```python
from build123d import *

# Parameters (mm, degrees)
SKETCH1_W           = 44.362146026
SKETCH1_H           = 10
BOSS_EXTRUDE1_DEPTH = 8
SKETCH2_R           = 1.6
CUT_EXTRUDE1_DEPTH  = 52.107729357
CUT_EXTRUDE2_START  = -17.925297
SKETCH3_R           = 3.05
CUT_EXTRUDE2_DEPTH  = 12.925297
FILLET1_R           = 2


with BuildPart() as part:
    # Sketch1 → Boss-Extrude1 (new body)
    with BuildSketch(Plane.XY):
        with BuildLine():
            Line((-29.953929645, -23), (-37.509998667, -23))
            ThreePointArc((-37.509998667, -23), (-35.812927639, -25.562359318), (-33.941125497, -28))
            Line((-33.941125497, -28), (-22.181073013, -28))
            Line((-22.181073013, -28), (-22.181073013, -23))
            Line((-22.181073013, -23), (-29.953929645, -23))
        make_face()
        with BuildLine():
            Line((-37.509998667, -23), (-43.266615306, -23))
            ThreePointArc((-43.266615306, -23), (0, -49), (43.266615306, -23))
            Line((43.266615306, -23), (37.509998667, -23))
            ThreePointArc((37.509998667, -23), (35.812927639, -25.562359318), (33.941125497, -28))
            ThreePointArc((33.941125497, -28), (28.503075122, -33.519765939), (22.181073013, -38))
            ThreePointArc((22.181073013, -38), (0, -44), (-22.181073013, -38))
            ThreePointArc((-22.181073013, -38), (-28.503075122, -33.519765939), (-33.941125497, -28))
            ThreePointArc((-33.941125497, -28), (-35.812927639, -25.562359318), (-37.509998667, -23))
        make_face()
        with BuildLine():
            Line((-22.181073013, -28), (-33.941125497, -28))
            ThreePointArc((-33.941125497, -28), (-28.503075122, -33.519765939), (-22.181073013, -38))
            Line((-22.181073013, -38), (-22.181073013, -28))
        make_face()
        with BuildLine():
            ThreePointArc((22.181073013, -38), (28.503075122, -33.519765939), (33.941125497, -28))
            Line((33.941125497, -28), (22.181073013, -28))
            Line((22.181073013, -28), (22.181073013, -38))
        make_face()
        with BuildLine():
            ThreePointArc((33.941125497, -28), (35.812927639, -25.562359318), (37.509998667, -23))
            Line((37.509998667, -23), (22.181073013, -23))
            Line((22.181073013, -23), (22.181073013, -28))
            Line((22.181073013, -28), (33.941125497, -28))
        make_face()
        with Locations((0, -33)):
            Rectangle(SKETCH1_W, SKETCH1_H)
        with BuildLine():
            Line((22.181073013, -38), (-22.181073013, -38))
            ThreePointArc((-22.181073013, -38), (0, -44), (22.181073013, -38))
        make_face()
    extrude(amount=BOSS_EXTRUDE1_DEPTH)

    # Sketch2 → Cut-Extrude1 (cut, through all)
    with BuildSketch(Plane(origin=(0, -23, 0), x_dir=(1, 0, 0), z_dir=(0, 1, 0))):
        with Locations(Location((-29.996615306, -4, 0), (0, 0, 270))):
            Circle(SKETCH2_R)
    cut_extrude1 = extrude(amount=-CUT_EXTRUDE1_DEPTH, mode=Mode.SUBTRACT)

    # Sketch3 → Cut-Extrude2 (cut)
    with BuildSketch(Plane(origin=(0, -23, 0), x_dir=(1, 0, 0), z_dir=(0, 1, 0)).offset(CUT_EXTRUDE2_START)):
        with Locations(Location((-29.996615306, -4, 0), (0, 0, 90))):
            Circle(SKETCH3_R)
    cut_extrude2 = extrude(amount=CUT_EXTRUDE2_DEPTH, mode=Mode.SUBTRACT)

    # Mirror1: Cut-Extrude1, Cut-Extrude2 across plane
    add(cut_extrude1.mirror(Plane(origin=(0, 0, 0), x_dir=(0, 0, 1), z_dir=(1, 0, 0))), mode=Mode.SUBTRACT)
    add(cut_extrude2.mirror(Plane(origin=(0, 0, 0), x_dir=(0, 0, 1), z_dir=(1, 0, 0))), mode=Mode.SUBTRACT)

    # Fillet1
    # the kernel refuses this fillet: 2 mm, written as the material it takes off along each edge
    with BuildSketch(Plane(origin=(22.181073013, -28, 8), x_dir=(0, -1, 0), z_dir=(-1, 0, 0))) as fillet1_piece_1:
        with BuildLine():
            CenterArc((FILLET1_R, -FILLET1_R), FILLET1_R, 90, 90)
            Line((0, -FILLET1_R), (0, 0))
            Line((0, 0), (FILLET1_R, 0))
        make_face()
    extrude(amount=44.362146026, mode=Mode.SUBTRACT)
    with BuildSketch(Plane(origin=(22.181073013, -28, 0), x_dir=(0, -1, 0), z_dir=(-1, 0, 0))) as fillet1_piece_2:
        with BuildLine():
            CenterArc((FILLET1_R, FILLET1_R), FILLET1_R, 180, 90)
            Line((0, FILLET1_R), (0, 0))
            Line((0, 0), (FILLET1_R, 0))
        make_face()
    extrude(amount=44.362146026, mode=Mode.SUBTRACT)
    with BuildSketch(Plane(origin=(22.181073013, -18, 0), x_dir=(1, 0, 0), z_dir=(0, -1, 0))) as fillet1_piece_3:
        with BuildLine():
            CenterArc((FILLET1_R, FILLET1_R), FILLET1_R, 180, 90)
            Line((0, FILLET1_R), (0, 0))
            Line((0, 0), (FILLET1_R, 0))
        make_face()
    extrude(amount=10, mode=Mode.SUBTRACT)
    with BuildSketch(Plane(origin=(-22.181073013, -28, 8), x_dir=(-1, 0, 0), z_dir=(0, 1, 0)), Plane(origin=(22.181073013, -18, 8), x_dir=(1, 0, 0), z_dir=(0, -1, 0)), Plane(origin=(-22.181073013, -28, 0), x_dir=(0, 0, 1), z_dir=(0, 1, 0))) as fillet1_piece_4:
        with BuildLine():
            CenterArc((FILLET1_R, -FILLET1_R), FILLET1_R, 90, 90)
            Line((0, -FILLET1_R), (0, 0))
            Line((0, 0), (FILLET1_R, 0))
        make_face()
    extrude(amount=10, mode=Mode.SUBTRACT)
    with BuildSketch(Plane(origin=(-17.181073013, -23, 8), x_dir=(0, -1, 0), z_dir=(-1, 0, 0)), Plane(origin=(48.266615306, -23, 8), x_dir=(0, -1, 0), z_dir=(-1, 0, 0)), Plane(origin=(-48.266615306, -23, 0), x_dir=(0, -1, 0), z_dir=(1, 0, 0))) as fillet1_piece_5:
        with BuildLine():
            CenterArc((FILLET1_R, -FILLET1_R), FILLET1_R, 90, 90)
            Line((0, -FILLET1_R), (0, 0))
            Line((0, 0), (FILLET1_R, 0))
        make_face()
    extrude(amount=31.085542293, mode=Mode.SUBTRACT)
    with BuildSketch(Plane(origin=(0, 0, 8), x_dir=(-0.9262421127905929, -0.3769291027411106, 0), z_dir=(-0.3769291027411106, 0.9262421127905929, 0))) as fillet1_piece_6:
        with BuildLine():
            CenterArc((49 - FILLET1_R, -FILLET1_R), FILLET1_R, 0, 90)
            Line((49, -FILLET1_R), (49, 0))
            Line((49, 0), (49 - FILLET1_R, 0))
        make_face()
    revolve(axis=Axis((0, 0, 8), (0, 0, 1)), revolution_arc=135.712813104, mode=Mode.SUBTRACT)
    with BuildSketch(Plane(origin=(48.266615306, -23, 0), x_dir=(0, -1, 0), z_dir=(-1, 0, 0))) as fillet1_piece_7:
        with BuildLine():
            CenterArc((FILLET1_R, FILLET1_R), FILLET1_R, 180, 90)
            Line((0, FILLET1_R), (0, 0))
            Line((0, 0), (FILLET1_R, 0))
        make_face()
    extrude(amount=31.085542293, mode=Mode.SUBTRACT)
    with BuildSketch(Plane(origin=(0, 0, 0), x_dir=(-0.9262421127905929, -0.3769291027411106, 0), z_dir=(-0.3769291027411106, 0.9262421127905929, 0))) as fillet1_piece_8:
        with BuildLine():
            CenterArc((49 - FILLET1_R, FILLET1_R), FILLET1_R, 270, 90)
            Line((49, FILLET1_R), (49, 0))
            Line((49, 0), (49 - FILLET1_R, 0))
        make_face()
    revolve(axis=Axis((0, 0, 0), (0, 0, 1)), revolution_arc=135.712813104, mode=Mode.SUBTRACT)
    with BuildSketch(Plane(origin=(22.181073013, -18, 8), x_dir=(1, 0, 0), z_dir=(0, -1, 0))) as fillet1_piece_9a_section:
        with BuildLine():
            CenterArc((FILLET1_R, -FILLET1_R), FILLET1_R, 90, 90)
            Line((0, -FILLET1_R), (0, 0))
            Line((0, 0), (FILLET1_R, 0))
        make_face()
    fillet1_piece_9a = extrude(amount=15, mode=Mode.PRIVATE)
    fillet1_piece_9a = split(fillet1_piece_9a, bisect_by=Plane(origin=(22.633863241, -28, 7.547209771), z_dir=(0, -1, 0)), keep=Keep.TOP, mode=Mode.PRIVATE)
    with BuildSketch(Plane(origin=(27.181073013, -28, 8), x_dir=(0, -1, 0), z_dir=(-1, 0, 0))) as fillet1_piece_9b_section:
        with BuildLine():
            CenterArc((FILLET1_R, -FILLET1_R), FILLET1_R, 90, 90)
            Line((0, -FILLET1_R), (0, 0))
            Line((0, 0), (FILLET1_R, 0))
        make_face()
    fillet1_piece_9b = extrude(amount=49.362146026, mode=Mode.PRIVATE)
    fillet1_piece_9b = split(fillet1_piece_9b, bisect_by=Plane(origin=(22.181073013, -28.452790229, 7.547209771), z_dir=(1, 0, 0)), keep=Keep.TOP, mode=Mode.PRIVATE)
    fillet1_piece_9 = fillet1_piece_9a & fillet1_piece_9b
    add(fillet1_piece_9, mode=Mode.SUBTRACT)
    with BuildSketch(Plane(origin=(22.181073013, -28, 8), x_dir=(0, -1, 0), z_dir=(-1, 0, 0))) as fillet1_piece_10a_section:
        with BuildLine():
            CenterArc((FILLET1_R, -FILLET1_R), FILLET1_R, 90, 90)
            Line((0, -FILLET1_R), (0, 0))
            Line((0, 0), (FILLET1_R, 0))
        make_face()
    fillet1_piece_10a = extrude(amount=49.362146026, mode=Mode.PRIVATE)
    fillet1_piece_10a = split(fillet1_piece_10a, bisect_by=Plane(origin=(-22.181073013, -28.452790229, 7.547209771), z_dir=(-1, 0, 0)), keep=Keep.TOP, mode=Mode.PRIVATE)
    with BuildSketch(Plane(origin=(-22.181073013, -33, 8), x_dir=(-1, 0, 0), z_dir=(0, 1, 0))) as fillet1_piece_10b_section:
        with BuildLine():
            CenterArc((FILLET1_R, -FILLET1_R), FILLET1_R, 90, 90)
            Line((0, -FILLET1_R), (0, 0))
            Line((0, 0), (FILLET1_R, 0))
        make_face()
    fillet1_piece_10b = extrude(amount=15, mode=Mode.PRIVATE)
    fillet1_piece_10b = split(fillet1_piece_10b, bisect_by=Plane(origin=(-22.633863241, -28, 7.547209771), z_dir=(0, -1, 0)), keep=Keep.TOP, mode=Mode.PRIVATE)
    fillet1_piece_10 = fillet1_piece_10a & fillet1_piece_10b
    add(fillet1_piece_10, mode=Mode.SUBTRACT)
    with BuildSketch(Plane(origin=(22.181073013, -18, 0), x_dir=(1, 0, 0), z_dir=(0, -1, 0))) as fillet1_piece_11a_section:
        with BuildLine():
            CenterArc((FILLET1_R, FILLET1_R), FILLET1_R, 180, 90)
            Line((0, FILLET1_R), (0, 0))
            Line((0, 0), (FILLET1_R, 0))
        make_face()
    fillet1_piece_11a = extrude(amount=15, mode=Mode.PRIVATE)
    fillet1_piece_11a = split(fillet1_piece_11a, bisect_by=Plane(origin=(22.633863241, -28, 0.452790229), z_dir=(0, -1, 0)), keep=Keep.TOP, mode=Mode.PRIVATE)
    with BuildSketch(Plane(origin=(27.181073013, -28, 0), x_dir=(0, -1, 0), z_dir=(-1, 0, 0))) as fillet1_piece_11b_section:
        with BuildLine():
            CenterArc((FILLET1_R, FILLET1_R), FILLET1_R, 180, 90)
            Line((0, FILLET1_R), (0, 0))
            Line((0, 0), (FILLET1_R, 0))
        make_face()
    fillet1_piece_11b = extrude(amount=49.362146026, mode=Mode.PRIVATE)
    fillet1_piece_11b = split(fillet1_piece_11b, bisect_by=Plane(origin=(22.181073013, -28.452790229, 0.452790229), z_dir=(1, 0, 0)), keep=Keep.TOP, mode=Mode.PRIVATE)
    fillet1_piece_11 = fillet1_piece_11a & fillet1_piece_11b
    add(fillet1_piece_11, mode=Mode.SUBTRACT)
    with BuildSketch(Plane(origin=(-22.181073013, -33, 0), x_dir=(0, 0, 1), z_dir=(0, 1, 0))) as fillet1_piece_12a_section:
        with BuildLine():
            CenterArc((FILLET1_R, -FILLET1_R), FILLET1_R, 90, 90)
            Line((0, -FILLET1_R), (0, 0))
            Line((0, 0), (FILLET1_R, 0))
        make_face()
    fillet1_piece_12a = extrude(amount=15, mode=Mode.PRIVATE)
    fillet1_piece_12a = split(fillet1_piece_12a, bisect_by=Plane(origin=(-22.633863241, -28, 0.452790229), z_dir=(0, -1, 0)), keep=Keep.TOP, mode=Mode.PRIVATE)
    with BuildSketch(Plane(origin=(22.181073013, -28, 0), x_dir=(0, -1, 0), z_dir=(-1, 0, 0))) as fillet1_piece_12b_section:
        with BuildLine():
            CenterArc((FILLET1_R, FILLET1_R), FILLET1_R, 180, 90)
            Line((0, FILLET1_R), (0, 0))
            Line((0, 0), (FILLET1_R, 0))
        make_face()
    fillet1_piece_12b = extrude(amount=49.362146026, mode=Mode.PRIVATE)
    fillet1_piece_12b = split(fillet1_piece_12b, bisect_by=Plane(origin=(-22.181073013, -28.452790229, 0.452790229), z_dir=(-1, 0, 0)), keep=Keep.TOP, mode=Mode.PRIVATE)
    fillet1_piece_12 = fillet1_piece_12a & fillet1_piece_12b
    add(fillet1_piece_12, mode=Mode.SUBTRACT)


solid = part.part
```
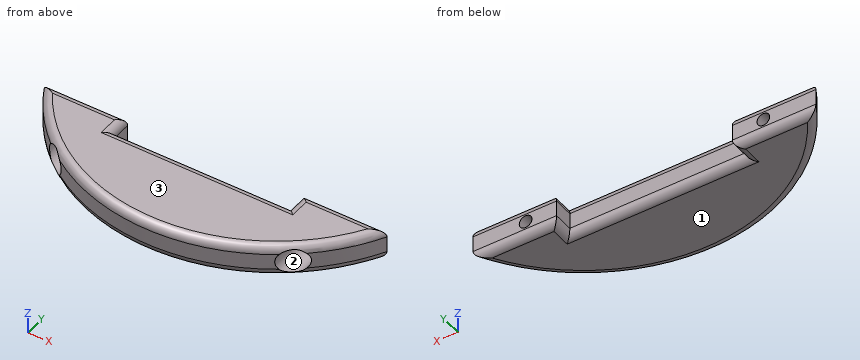
Part model, mm, in its own coordinate system. Face numbers are marked on the shaded views. Round coordinates to 2 decimals unless told otherwise and drop trailing zeros. Loops run counter-clockwise (first coordinate to the right, second up) from the corner with the lowest first, then second, coordinate; pieces in that order, holes last. Notation, with made-up numbers: (-29, -37.75) -> (10, -37.75) arc R23 cw to (10, -15.75) -> close; hole circle Ø2 at (-22.5, -20.75). An arc over 180 degrees is marked (long way). Use a Markdown table: item, result.
1) Cut at B-B, the plane y = -27. State how many separate pieces and enclosed holes the cut face has, and give its area (3 significant figures).
The answers:
| item | result |
|---|---|
| separate pieces | 2 |
| enclosed holes | 2 |
| area | 276 mm2 |
2) Probe line 1 (X direction, y = -33.25, z = 5); line 2 (X direction, y = -24.2, z = 4); line 3 (Y direction, x = 1, z = 3.5). List the from-to ranges inside material, lowest first. Write a range as [from, to].
The answers:
| item | result |
|---|---|
| line 1 | x = [-35.99, -32.88], [-27.12, 27.12], [32.88, 35.99] |
| line 2 | x = [-42.61, -31.6], [-28.4, -22.18], [22.18, 28.4], [31.6, 42.61] |
| line 3 | y = [-48.99, -28] |
3) Pull direction Z, two halves, no side cores. Call the marked faces 1, 2 and 3: pulls with the +Z half, pulls with the -Z half, needs draft (parallel to the pull), parting line crosses it, or undercut.
The answers:
| item | result |
|---|---|
| face 1 | pulls with the -Z half |
| face 2 | undercut |
| face 3 | pulls with the +Z half |
4) Cut at A-A, the plane z = 4.5. List the corners of the cut face in (x, y), and give its area (3 significant figures).
The answers:
| item | result |
|---|---|
| outline | (-43.27, -23) arc R49 ccw to (-33.01, -36.22) -> (-33.01, -28) -> (-31.52, -28) -> (-31.52, -23) -> close; (-28.48, -28) -> (-26.99, -28) -> (-26.99, -40.9) arc R49 ccw to (26.99, -40.9) -> (26.99, -28) -> (28.48, -28) -> (28.48, -23) -> (22.18, -23) -> (22.18, -28) -> (-22.18, -28) -> (-22.18, -23) -> (-28.48, -23) -> close; (31.52, -28) -> (33.01, -28) -> (33.01, -36.22) arc R49 ccw to (43.27, -23) -> (31.52, -23) -> close |
| area | 1,220 mm2 |
5) Drop flat-ended pins along their axis: pin 1 Ø1.9 at (x, z) = (30, 4) entering from +Y; pin 2 Ø1.2 at (y, z) = (-26, 4) entering from -X; pin 3 Ø1.5 at (x, z) = (14.5, 7) entering from +Y; pin 4 Ø3.5 at (x, z) = (-30, 4) entering from -Y. Give the stop position or say it passes through.
The answers:
| item | result |
|---|---|
| pin 1 | passes through |
| pin 2 | stops at x = -41.9 |
| pin 3 | stops at y = -28.02 |
| pin 4 | stops at y = -28 |
